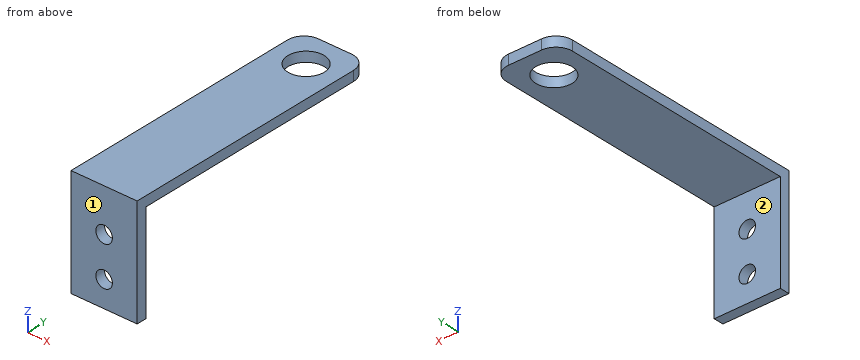
Autodesk Inventor part; units mm, degrees
ref_plane "YZ Plane" through (0, 0, 0) normal (1, 0, 0) x (0, 1, 0)
ref_plane "XZ Plane" through (0, 0, 0) normal (0, 1, 0) x (-1, 0, 0)
ref_plane "XY Plane" through (0, 0, 0) normal (0, 0, 1) x (1, 0, 0)
sketch "Sketch1" plane through (0, 0, 0) normal (0, 0, 1) x (1, 0, 0)
  line L0 (0, 0) -> (20, 0)
  line L1 (20, 0) -> (20, 80)
  line L2 (20, 80) -> (0, 80)
  line L3 (0, 80) -> (0, 0)
  circle A0 centre (10, 70) radius 5.5
  line L4 (20, 0) -> (0, 0)
  line L5 (0, 0) -> (0, 3)
  line L6 (0, 3) -> (20, 3)
  line L7 (20, 3) -> (20, 0)
  point P0 (10, 0)
  dimension "d0" = 20
  dimension "d1" = 80
  dimension "d2" = 11
  dimension "d3" = 70
  dimension "d7" = 3
extrude "Extrusion1" add sketch "Sketch1" along normal blind 3
fillet "Fillet1" radius 5 2 edges at (20, 80, 1.5) (0, 80, 1.5)
extrude "Extrusion2" add sketch "Sketch1" against normal blind 30 contours L3 L6 L1 L0
sketch "Sketch2" plane through (0, 3, 0) normal (0, 1, 0) x (1, 0, 0)
  circle A0 centre (10, 22.1006) radius 2.5
  circle A1 centre (10, 10.048) radius 2.5
  point P0 (0, 0)
  dimension "d10" = 5
  dimension "d11" = 5
extrude "Extrusion3" cut sketch "Sketch2" against normal through all
extrude "Extrusion4" cut sketch "Sketch1" along normal blind 10 contours A0
extrude "Extrusion5" cut sketch "Sketch1" along normal blind 10 contours A0
properties part number "roll stand"
Source: CAD feature listing. Evaluate the final solid. Frame: model axes, mm. Face numbers are marked on the shaded views. A direction names the side the tool comes from. Give positions to 0.01 mm unless a question says otherwise; leave off trailing zeros. Loops run counter-clockwise (first coordinate to the right, second up) from the corner with the lowest first, then second, coordinate; pieces in that order, holes last. Notation, with made-up numbers: (2, 50) -> (50, 50) arc R26 cw to (50, 72) -> close; hole circle Ø3 at (-11.75, 64). An arc over 180 degrees is marked (long way). Use a Markdown table: item, result. Add a question column.
(1) Section query B-B (x = 10). Output: boundary loops of the cut face in (y, z).
(2) Section query D-D (z = -27). Output: boundary loops of the cut face in (x, y), then the cut area to 3 significant figures.
(3) Section query A-A (y = 70). Output: boundary loops of the cut face in (x, z), then the cut area to 3 significant figures.
(4) First-contact query: pin 1 Ø1.5 at (x, z) = (16.5, -7.5) entering from +Y; pin 2 Ø6.5 at (x, y) = (10, 70) entering from +Z; pin 3 Ø6 at (x, y) = (10.5, 53) entering from -Z. Flat tips, straight axial feed; report the tip coordinate or a pass-through.
(5) Access query for the marked faces 1 and 2. Directions: +Z, -Z, +X, -X, +Y, -Y. A direction counts if a zero-diameter tool reaches every point of the face in a straight line with its end or side. Return the directions, or none.
(6) Section query C-C (z = -23.5). Output: boundary loops of the cut face in (x, y).
(7) Ray query, line 1 (Z direction, x = 10, y = 0.95); line 2 (Y direction, x = 10, z = 1.7); line 3 (Y direction, x = 12, z = -13.5). Return the intervals inside material, ascending.
Checked values:
| question | item | result |
|---|---|---|
| 1 | outline | (0, -30) -> (3, -30) -> (3, -24.6) -> (0, -24.6) -> close; (0, -19.6) -> (3, -19.6) -> (3, -12.55) -> (0, -12.55) -> close; (0, -7.55) -> (3, -7.55) -> (3, 0) -> (64.5, 0) -> (64.5, 3) -> (0, 3) -> close; (75.5, 0) -> (80, 0) -> (80, 3) -> (75.5, 3) -> close |
| 2 | outline | (0, 0) -> (20, 0) -> (20, 3) -> (0, 3) -> close |
| 2 | area | 60.0 mm^2 |
| 3 | outline | (0, 0) -> (4.5, 0) -> (4.5, 3) -> (0, 3) -> close; (15.5, 0) -> (20, 0) -> (20, 3) -> (15.5, 3) -> close |
| 3 | area | 27.0 mm^2 |
| 4 | pin 1 | y = 3 |
| 4 | pin 2 | through |
| 4 | pin 3 | z = 0 |
| 5 | face 1 | +Z, -Z, +X, -X, -Y |
| 5 | face 2 | -Z, +X, -X, +Y |
| 6 | outline | (0, 0) -> (7.93, 0) -> (7.93, 3) -> (0, 3) -> close; (12.07, 0) -> (20, 0) -> (20, 3) -> (12.07, 3) -> close |
| 7 | line 1 | -30 to -24.6, -19.6 to -12.55, -7.55 to 3 |
| 7 | line 2 | 0 to 64.5, 75.5 to 80 |
| 7 | line 3 | 0 to 3 |
